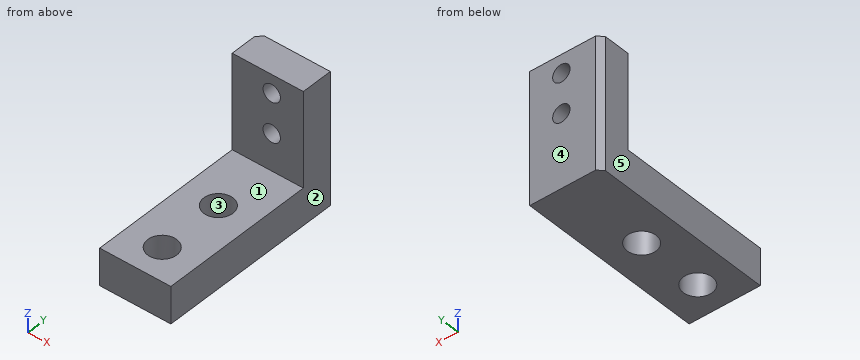
from build123d import *

# Parameters (mm, degrees)
SKETCH1_W             = 13.5
SKETCH1_H             = 35.5
SKETCH1_R             = 2.75
BOSS_EXTRUDE1_DEPTH   = 7
SKETCH2_W             = 13.5
SKETCH2_H             = 6
BOSS_EXTRUDE2_DEPTH   = 18
CHAMFER1_SIZE         = 1
M4X0_7_TAPPED_HOLE1_D = 3.3


with BuildPart() as part:
    # Sketch1 → Boss-Extrude1 (new body)
    with BuildSketch(Plane.XY):
        with Locations((-10.919683258, -1.606334842)):
            Rectangle(SKETCH1_W, SKETCH1_H)
        with Locations((-10.919683258, -13.356334842)):
            Circle(SKETCH1_R, mode=Mode.SUBTRACT)
        with Locations((-10.919683258, -0.856334842)):
            Circle(SKETCH1_R, mode=Mode.SUBTRACT)
    extrude(amount=BOSS_EXTRUDE1_DEPTH)

    # Sketch2 → Boss-Extrude2 (add)
    with BuildSketch(Plane.XY.offset(7)):
        with Locations((-10.919683258, 13.143665158)):
            Rectangle(SKETCH2_W, SKETCH2_H)
    extrude(amount=BOSS_EXTRUDE2_DEPTH)

    # Chamfer1
    chamfer1_edges = [part.edges().sort_by_distance(p)[0] for p in [
        (-17.669683258, 16.143665158, 12.5),
    ]]
    chamfer(chamfer1_edges, length=CHAMFER1_SIZE)

    # M4x0.7 Tapped Hole1 (through all)
    with Locations(Plane(origin=(0, 16.143665158, 0), x_dir=(1, 0, 0), z_dir=(0, 1, 0))):
        with Locations((-10.169683258, -21.5), (-10.169683258, -14)):
            Hole(M4X0_7_TAPPED_HOLE1_D / 2)


solid = part.part
Input: part model. Units: mm. Frame: model coordinates. Face numbers are marked on the shaded views. A direction names the side the tool comes from. Coordinates: 2 decimals unless noted, no trailing zeros. Loops run counter-clockwise (first coordinate to the right, second up) from the corner with the lowest first, then second, coordinate; pieces in that order, holes last. Notation, with made-up numbers: (23.5, -11.5) -> (60.5, -11.5) arc R19 cw to (60.5, 13.5) -> close; hole circle Ø4 at (52, 47). An arc over 180 degrees is marked (long way). One line per item, written item: value.
(1) Set-up query: the marked faces 1 and 2. Return all of +Z, -Z, +X, -X, +Y, -Y with unobstructed straight access to the full face (end or side cutting, diameter ignored); none if empty.
Answer below:
face 1: +Z, +X, -X, -Y
face 2: +Z, -Z, +X, +Y, -Y
(2) Ray query, line 1 along Z through (x, y) = (-13.5, 3); line 2 along Y through (x, z) = (-12.5, 22.5); line 3 along X through (y, z) = (11.5, 23). Return the intervals inside material, ascending.
Answer below:
line 1: z = 0 to 7
line 2: y = 10.14 to 16.14
line 3: x = -17.67 to -10.86, -9.48 to -4.17
(3) Cut plane D-D (z = 6). Output: boundary loops of the cut face in (x, y), then the cut area to 3 significant figures.
Answer below:
outline: (-17.67, -19.36) -> (-4.17, -19.36) -> (-4.17, 16.14) -> (-16.67, 16.14) -> (-17.67, 15.14) -> close; hole circle Ø5.5 at (-10.92, -13.36); hole circle Ø5.5 at (-10.92, -0.86)
area: 431 mm2
(4) Pin query (flat end, axial travel): pin 1 Ø2 at (x, y) = (-7.5, 9) entering from -Z; pin 2 Ø2 at (x, z) = (-16, 10.5) entering from -Y; pin 3 Ø6 at (x, y) = (-5.5, -15) entering from +Z. Return the tip coordinate at first contact, or that it passes through.
Answer below:
pin 1: stops at z = 0
pin 2: stops at y = 10.14
pin 3: stops at z = 7
(5) Cut plane B-B (x = -12.25). Output: boundary loops of the cut face in (y, z), then the cut area to 3 significant figures.
Answer below:
outline: (-19.36, 0) -> (-15.76, 0) -> (-15.76, 7) -> (-19.36, 7) -> close; (-10.95, 0) -> (-3.26, 0) -> (-3.26, 7) -> (-10.95, 7) -> close; (1.55, 0) -> (16.14, 0) -> (16.14, 25) -> (10.14, 25) -> (10.14, 7) -> (1.55, 7) -> close
area: 289 mm2
(6) Cut plane C-C (y = -15.5). Output: boundary loops of the cut face in (x, z), then the cut area to 3 significant figures.
Answer below:
outline: (-17.67, 0) -> (-12.64, 0) -> (-12.64, 7) -> (-17.67, 7) -> close; (-9.2, 0) -> (-4.17, 0) -> (-4.17, 7) -> (-9.2, 7) -> close
area: 70.4 mm2
(7) Draft query along Y for the marked faces 3, 4 and 5. Return one class per face: pulls with the +Y half, pulls with the -Y half, needs draft (parallel to the pull), parting line crosses it, or undercut.
Answer below:
face 3: undercut
face 4: pulls with the +Y half
face 5: needs draft
(8) Cut plane A-A (z = 21.5). Output: boundary loops of the cut face in (x, y), then the cut area to 3 significant figures.
Answer below:
outline: (-17.67, 10.14) -> (-11.82, 10.14) -> (-11.82, 16.14) -> (-16.67, 16.14) -> (-17.67, 15.14) -> close; (-8.52, 10.14) -> (-4.17, 10.14) -> (-4.17, 16.14) -> (-8.52, 16.14) -> close
area: 60.7 mm2
